Design review of the part built by this model. Coordinates are the model's own, in mm. A direction names the side the tool comes from. Coordinates: 2 decimals unless noted, no trailing zeros. Loops run counter-clockwise (first coordinate to the right, second up) from the corner with the lowest first, then second, coordinate; pieces in that order, holes last. Notation, with made-up numbers: (63.5, 0) -> (117.5, 0) arc R16 ccw to (117.5, 22) -> close; hole circle Ø9 at (60.5, -10.5). An arc over 180 degrees is marked (long way). One line per item, written item: value. Start each with the question number.
1. Add section C-C on y = 20.5. Write out the cut boundary in (x, z).
2. Draft analysis for pull direction Z (two halves, no side actions). For faces 4 (the flat face through (-84, 19, 60.946)), 5 (the flat face through (-53.874, 19, 34)), 6 (the flat face through (-84, 29, 7.946)), state which applies: pulls with the +Z half, pulls with the -Z half, needs draft (parallel to the pull), parting line crosses it, or undercut.
3. Add section D-D on x = -68.5. Write out the cut boundary in (y, z), plus the area to 3 significant figures.
4. Add section A-A on x = -107.5. Write out the cut boundary in (y, z), plus the area to 3 significant figures.
5. Insertion check: pin 1 (10 mm diameter, centred on x = -105.5, z = 23.5, fed in from -Y); pin 2 (0.5 mm diameter, centred on x = -99, z = 44.5, fed in from +Y); pin 3 (6.5 mm diameter, centred on x = -107.5, z = 43, fed in from +Y). Each pin has a flat end and moves straight along its axis. Give the tip position at first contact, or say it passes through.
6. For probe 1 along X at (y, z) = (20.5, 38.5); probe 2 along Z at (x, y) = (-84, 25.5); probe 3 along X at (y, z) = (14, 23), list the stretches that pass through material, from the lowest coordinate up.
7. Machinability: for faces 1 (the flat face through (-95, 9, 59.946)), 2 (the flat face through (-98.874, 21, 34)), 3 (the flat face through (-71, 0, 34)), which of the approach directions +Z, -Z, +X, -X, +Y, -Y give a long, thin tool a straight path to every point of the face, cutting with its end or side? Answer none if there is none.
8. Add section B-B on y = 10.5. Write out the cut boundary in (x, z), plus the area to 3 significant figures.
```python
from build123d import *

# Parameters (mm, degrees)
SKETCH1_W           = 60
SKETCH1_H           = 54
BOSS_EXTRUDE1_DEPTH = 38
SKETCH2_W           = 44
SKETCH2_H           = 52
CUT_EXTRUDE1_DEPTH  = 19
SKETCH3_W           = 35
SKETCH3_H           = 52
CUT_EXTRUDE2_DEPTH  = 18
SKETCH4_W           = 6
SKETCH4_H           = 10
CUT_EXTRUDE3_DEPTH  = 38
SKETCH5_W           = 14
SKETCH5_H           = 52
CUT_EXTRUDE5_DEPTH  = 15
SKETCH6_W           = 13
SKETCH6_H           = 52
CUT_EXTRUDE6_DEPTH  = 4


with BuildPart() as part:
    # Sketch1 → Boss-Extrude1 (new body)
    with BuildSketch(Plane(origin=(0, 0, 0), x_dir=(1, 0, 0), z_dir=(0, 1, 0))):
        with Locations((-83.874465942, -33.946435202)):
            Rectangle(SKETCH1_W, SKETCH1_H)
    extrude(amount=BOSS_EXTRUDE1_DEPTH)

    # Sketch2 → Cut-Extrude1 (cut)
    with BuildSketch(Plane(origin=(0, 38, 0), x_dir=(1, 0, 0), z_dir=(0, 1, 0))):
        with Locations((-76.874465942, -33.946435202)):
            Rectangle(SKETCH2_W, SKETCH2_H)
    extrude(amount=-CUT_EXTRUDE1_DEPTH, mode=Mode.SUBTRACT)

    # Sketch3 → Cut-Extrude2 (cut)
    with BuildSketch(Plane(origin=(0, 0, 0), x_dir=(-1, 0, 0), z_dir=(0, -1, 0))):
        with Locations((95.374465942, -33.946435202)):
            Rectangle(SKETCH3_W, SKETCH3_H)
    extrude(amount=-CUT_EXTRUDE2_DEPTH, mode=Mode.SUBTRACT)

    # Sketch4 → Cut-Extrude3 (cut)
    with BuildSketch(Plane(origin=(0, 18, 0), x_dir=(-1, 0, 0), z_dir=(0, -1, 0))):
        with Locations((108.874465942, -34.946435202)):
            Rectangle(SKETCH4_W, SKETCH4_H)
    extrude(amount=-CUT_EXTRUDE3_DEPTH, mode=Mode.SUBTRACT)

    # Sketch5 → Cut-Extrude5 (cut)
    with BuildSketch(Plane(origin=(0, 38, 0), x_dir=(1, 0, 0), z_dir=(0, 1, 0))):
        with Locations((-105.874465942, -33.946435202)):
            Rectangle(SKETCH5_W, SKETCH5_H)
    extrude(amount=-CUT_EXTRUDE5_DEPTH, mode=Mode.SUBTRACT)

    # Sketch6 → Cut-Extrude6 (cut)
    with BuildSketch(Plane(origin=(0, 23, 0), x_dir=(1, 0, 0), z_dir=(0, 1, 0))):
        with Locations((-106.374465942, -33.946435202)):
            Rectangle(SKETCH6_W, SKETCH6_H)
    extrude(amount=-CUT_EXTRUDE6_DEPTH, mode=Mode.SUBTRACT)


solid = part.part
```
Worked answers:
1. outline: (-113.87, 6.95) -> (-53.87, 6.95) -> (-53.87, 60.95) -> (-113.87, 60.95) -> close; hole (-112.87, 7.95) -> (-99.87, 7.95) -> (-99.87, 59.95) -> (-112.87, 59.95) -> close; hole (-98.87, 7.95) -> (-54.87, 7.95) -> (-54.87, 59.95) -> (-98.87, 59.95) -> close
2. face 4: pulls with the +Z half
2. face 5: needs draft
2. face 6: undercut
3. outline: (0, 6.95) -> (38, 6.95) -> (38, 7.95) -> (19, 7.95) -> (19, 59.95) -> (38, 59.95) -> (38, 60.95) -> (0, 60.95) -> close
3. area: 1,060 mm²
4. outline: (0, 6.95) -> (38, 6.95) -> (38, 7.95) -> (19, 7.95) -> (19, 29.95) -> (18, 29.95) -> (18, 7.95) -> (0, 7.95) -> close; (0, 59.95) -> (18, 59.95) -> (18, 39.95) -> (19, 39.95) -> (19, 59.95) -> (38, 59.95) -> (38, 60.95) -> (0, 60.95) -> close
4. area: 118 mm²
5. pin 1: stops at y = 18
5. pin 2: stops at y = 23
5. pin 3: stops at y = 19
6. probe 1: x = -113.87 to -112.87, -99.87 to -98.87, -54.87 to -53.87
6. probe 2: z = 6.95 to 7.95, 59.95 to 60.95
6. probe 3: x = -113.87 to -112.87, -77.87 to -53.87
7. face 1: -Y
7. face 2: +Y
7. face 3: +Z, -Z, +X, -X, -Y
8. outline: (-113.87, 6.95) -> (-53.87, 6.95) -> (-53.87, 60.95) -> (-113.87, 60.95) -> close; hole (-112.87, 7.95) -> (-77.87, 7.95) -> (-77.87, 59.95) -> (-112.87, 59.95) -> close
8. area: 1,420 mm²
